Part model, mm, in its own coordinate system. A direction names the side the tool comes from. Give positions to 0.01 mm unless a question says otherwise; leave off trailing zeros. Write each loop counter-clockwise with the first axis right and the second up, starting at its lowest first coordinate (ties: lowest second). Pieces come first, ordered by that corner, then holes. Notation, with made-up numbers: M -39,82.5 L -6,82.5 A28 ccw -6,120.5 Z; hole C 32,-10 d11. An arc over 180 degrees is marked long. Write item = value, one per line. Start each with the question number.
from build123d import *

# Parameters (mm, degrees)
BOSS_EXTRUDE1_DEPTH     = 26.5
CHAMFER1_START          = -5.68864596
CHAMFER1_OUTLINE_W      = 26.5
CHAMFER1_OUTLINE_H      = 7
CHAMFER1_DEPTH          = 3.235738337
CUT_EXTRUDE1_DEPTH      = 33.870959828
CUT_EXTRUDE1_DEPTH_BACK = 33.870959828


with BuildPart() as part:
    # Sketch1 → Boss-Extrude1 (new body)
    with BuildSketch(Plane(origin=(0, 0, 0), x_dir=(0, 0, -1), z_dir=(1, 0, 0))):
        with BuildLine():
            Line((-2, 9.25), (-3, 9.25))
            ThreePointArc((-3, 9.25), (-5.121320344, 8.371320344), (-6, 6.25))
            Line((-6, 6.25), (-6, -6.25))
            ThreePointArc((-6, -6.25), (-5.121320344, -8.371320344), (-3, -9.25))
            Line((-3, -9.25), (6, -9.25))
            Line((6, -9.25), (6, -7.75))
            Line((6, -7.75), (4, -7.75))
            ThreePointArc((4, -7.75), (-0.242640687, -5.992640687), (-2, -1.75))
            Line((-2, -1.75), (-2, 9.25))
        make_face()
    extrude(amount=BOSS_EXTRUDE1_DEPTH)

    # Chamfer1: read off the stored shape, not the designer's step
    # Chamfer1 outline → Chamfer1 (cut)
    with BuildSketch(Plane(origin=(0, 0, 0), x_dir=(1, 0, 0), z_dir=(0, 0.897390589003635, -0.441237046005556)).offset(CHAMFER1_START)):
        with Locations((13.25, 7.5)):
            Rectangle(CHAMFER1_OUTLINE_W, CHAMFER1_OUTLINE_H)
    extrude(amount=CHAMFER1_DEPTH, mode=Mode.SUBTRACT)

    # Sketch2 → Cut-Extrude1 (cut, two sides: drawn at the far end of the back side and taken through both)
    with BuildSketch(Plane.XZ.offset(9.25).offset(-CUT_EXTRUDE1_DEPTH_BACK)):
        Polygon((23.85, -5.920212303), (26.5, -5.920212303), (25.175, -3.625244983), align=None)
        Polygon((21.2, -5.920212303), (23.85, -5.920212303), (22.525, -3.625244983), align=None)
        Polygon((18.55, -5.920212303), (21.2, -5.920212303), (19.875, -3.625244983), align=None)
        Polygon((15.9, -5.920212303), (18.55, -5.920212303), (17.225, -3.625244983), align=None)
        Polygon((13.25, -5.920212303), (15.9, -5.920212303), (14.575, -3.625244983), align=None)
        Polygon((10.6, -5.920212303), (13.25, -5.920212303), (11.925, -3.625244983), align=None)
        Polygon((7.95, -5.920212303), (10.6, -5.920212303), (9.275, -3.625244983), align=None)
        Polygon((5.3, -5.920212303), (7.95, -5.920212303), (6.625, -3.625244983), align=None)
        Polygon((2.65, -5.920212303), (5.3, -5.920212303), (3.975, -3.625244983), align=None)
        Polygon((2.65, -5.920212303), (1.325, -3.625244983), (0, -5.920212303), align=None)
    extrude(amount=CUT_EXTRUDE1_DEPTH + CUT_EXTRUDE1_DEPTH_BACK, mode=Mode.SUBTRACT)


solid = part.part
Q1. Slice it at D-D (z = -4.75). Give the number of separate pieces and of enclosed holes in the cut face, and give its area (3 significant figures).
Q2. Two-plate mould, pull along X, no slides. Class faces 1 (the face through (0, -2, 3)), 2 (the face through (22.902, -8.929, -4.279)), 3 (the face through (13.06, -8.35, 5.14)): +X half, -X half, draft (parallel to the pull), parting line (faces both ways), or undercut.
Q3. Probe line 1 along Z through (x, y) = (14.5, 0.25); line 2 along Z through (x, y) = (18.5, -5); line 3 along Y through (x, z) = (4.5, -3). List the from-to ranges inside material, lowest first.
Q4. Slice it at B-B (y = 1.5). Give the cut face in (x, z).
Q5. Drop a flat-ended pin along its axis: P1, Ø10, axis at x = 6, y = 4.5, coming from the -Z side. Give the stop position or say it passes through.
Q6. Tool access for faces 4 (the face through (8.916, -8.929, -4.247)), 5 (the face through (13, 0, 6)): list every direction of +Z, -Z, +X, -X, +Y, -Y with a clear straight run to the whole face (end or side of a thin tool).
Q7. Slice it at A-A (x = 10). Give the cut face in (y, z), and give its area (3 significant figures).
Q8. Slice it at C-C (z = 5.5). Give the cut face in (x, y).
Working result:
q1.separate_pieces = 11
q1.enclosed_holes = 0
q1.area = 7.77 mm2
q2.face_1 = -X half
q2.face_2 = undercut
q2.face_3 = draft
q3.line_1 = 2 to 6
q3.line_2 = 1.04 to 6
q3.line_3 = -9.25 to -7.81
q4.outline = M 0,2 L 26.5,2 L 26.5,6 L 0,6 Z
q5.P1 = 2
q6.face_4 = -Z, +Y, -Y
q6.face_5 = +Z, +X, -X, +Y, -Y
q7.outline = M -9.25,-4.88 L -8.74,-4.88 L -7.55,-2.46 A6 cw -1.75,2 L 9.25,2 L 9.25,3 A3 ccw 6.25,6 L -6.25,6 A3 ccw -9.25,3 Z
q7.area = 87.1 mm2
q8.outline = M 0,-7.91 L 26.5,-7.91 L 26.5,7.91 L 0,7.91 Z
